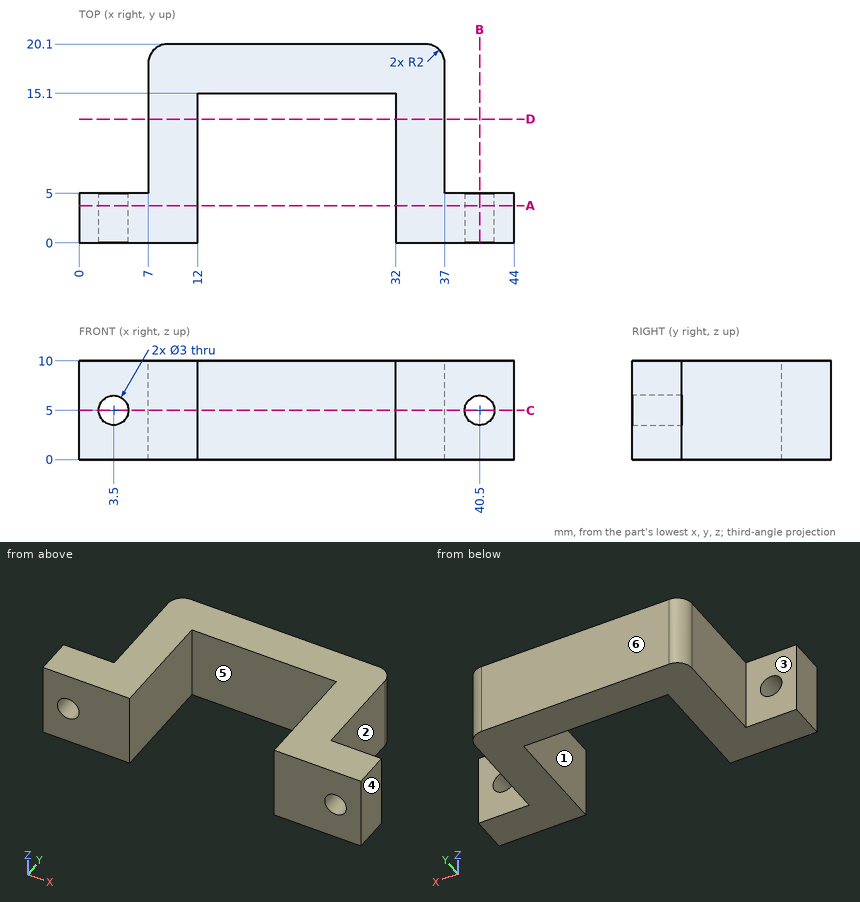
Job drawing, mm, ordinate dimensions from the low corner. One solid piece. A direction names the side the tool comes from. Coordinates: 2 decimals unless noted, no trailing zeros. Order: outer loops, then holes, each group sorted by start corner. A loop starts at its lowest first (then second) coordinate and runs counter-clockwise, first axis right, second up. Notation, with made-up numbers: (65, 66.25) - (89, 66.25) arc R15 ccw to (89, 94.25) - close; hole circle Ø8 at (82, 50.5). An arc over 180 degrees is marked (long way). Return JSON: item names as keys, results as strings. Group by question number.
1) Saw through at A-A, the plane y = 3.75. Write the cut outline in (x, z), plus the area to 3 significant figures.
2) Saw through at B-B, the plane x = 40.5. Write the cut outline in (y, z).
3) Saw through at C-C, the plane z = 5. Write the cut outline in (x, y).
4) Probe line 1 (X direction, y = 13.75, z = 5); line 2 (Z direction, x = 40.5, y = 1.5); line 3 (Y direction, x = 19, z = 8.5). List the from-to ranges inside material, lowest first. Write a range as from..to.
5) Flat gauge pins, fed straight in: P1, Ø4, axis at y = 13.5, z = 9, coming from the +X side; P2, Ø5.5, axis at x = 2.5, z = 4.5, coming from the +Y side; P3, Ø1.8, axis at x = 3.5, z = 5, coming from the +Y side. Where does each tip first touch, or does it go through?
6) Mould opens along X. For the marked faces 4, 5 and 6 say: released by +X, released by -X, zero draft, split by the parting line, or undercut.
7) Saw through at D-D, the plane y = 12.5. Write the cut outline in (x, z).
8) Tool access for the marked faces 1, 2 and 3: list every direction of +Z, -Z, +X, -X, +Y, -Y with a clear straight run to the whole face (end or side of a thin tool).
Values found:
{
 "1": {"outline": "(0, 0) - (12, 0) - (12, 10) - (0, 10) - close; (32, 0) - (44, 0) - (44, 10) - (32, 10) - close; hole circle Ø3 at (3.5, 5); hole circle Ø3 at (40.5, 5)", "area": "226 mm²"},
 "2": {"outline": "(0, 0) - (5, 0) - (5, 3.5) - (0, 3.5) - close; (0, 6.5) - (5, 6.5) - (5, 10) - (0, 10) - close"},
 "3": {"outline": "(0, 0) - (2, 0) - (2, 5) - (0, 5) - close; (5, 0) - (12, 0) - (12, 15.1) - (32, 15.1) - (32, 0) - (39, 0) - (39, 5) - (37, 5) - (37, 18.1) arc R2 ccw to (35, 20.1) - (9, 20.1) arc R2 ccw to (7, 18.1) - (7, 5) - (5, 5) - close; (42, 0) - (44, 0) - (44, 5) - (42, 5) - close"},
 "4": {"line 1": "x = 7..12, 32..37", "line 2": "z = 0..3.5, 6.5..10", "line 3": "y = 15.1..20.1"},
 "5": {"P1": "stops at x = 37", "P2": "stops at y = 5", "P3": "passes through"},
 "6": {"face 4": "released by +X", "face 5": "undercut", "face 6": "zero draft"},
 "7": {"outline": "(7, 0) - (12, 0) - (12, 10) - (7, 10) - close; (32, 0) - (37, 0) - (37, 10) - (32, 10) - close"},
 "8": {"face 1": "+Z, -Z, -Y", "face 2": "+Z, -Z, +X, +Y", "face 3": "+Z, -Z, -X, +Y"}
}
